For this review, take the finished solid that the model builds, in its own axes (mm). A direction names the side the tool comes from. Give positions to 0.01 mm unless a question says otherwise; leave off trailing zeros. Order: outer loops, then holes, each group sorted by start corner. A loop starts at its lowest first (then second) coordinate and runs counter-clockwise, first axis right, second up. Notation, with made-up numbers: (68.5, 9.5) - (94.5, 9.5) arc R31 ccw to (94.5, 44.5) - close; hole circle Ø7 at (35.25, 86.5). An arc over 180 degrees is marked (long way). Use a Markdown table: item, result. Add a question column.
1) Machinability: for faces 1 (the face through (3.451, 1.521, -6.645)), 2 (the face through (4, 0.8, -3)), which of the approach directions +Z, -Z, +X, -X, +Y, -Y give a long, thin tool a straight path to every point of the face, cutting with its end or side? Answer none if there is none.
2) We need section A-A on y = 2.7. Give the number of separate pieces and of enclosed holes in the cut face, then the cut area to 3 significant figures.
3) Clearance check with flat-ended pins moving along their axes: P1, Ø1.5, axis at y = 1, z = -6, coming from the -X side; P2, Ø2, axis at x = 3.5, z = -3.5, coming from the -Y side; P3, Ø1, axis at x = 4, y = 2.5, coming from the -Z side. State where each tip first meets the part, or that it passes through.
4) Wall thickness on L1, parallel to Y at x = 3, z = -3; L2, parallel to X at y = 0.3, z = -3.5; L3, parallel to X at y = 0.6, z = -4: over which ranges is each line inside the solid? List them lowest first.
5) We need section B-B on y = 0.45. Write out the cut boundary in (x, z) (3 decimals), then the cut area to 3 significant figures.
6) We need section C-C on z = -1.25. Write out the cut boundary in (x, y).
7) Mouldability with a two-part tool opening along X and no side actions: class faces 3 (the face through (2, 0, -5)), 4 (the face through (6.655, 1.479, -3.451)), 5 (the face through (4.041, 0.394, -5.217)), 6 (the face through (3.9, 2.6, -2.68)) as released by +X, released by -X, zero draft, split by the parting line, or undercut.
8) We need section D-D on y = 1.65. Write out the cut boundary in (x, z) (3 decimals), then the cut area to 3 significant figures.
```python
from build123d import *

# Parameters (mm, degrees)
SKETCH1_W           = 7
SKETCH1_H           = 7
BOSS_EXTRUDE1_DEPTH = 3
CUT_EXTRUDE1_DEPTH  = 7
CUT_EXTRUDE2_DEPTH  = 11
SKETCH4_R           = 1.8
CUT_EXTRUDE3_DEPTH  = 0.8
CUT_EXTRUDE4_DEPTH  = 0.4


with BuildPart() as part:
    # Sketch1 → Boss-Extrude1 (new body)
    with BuildSketch(Plane(origin=(0, 0, 0), x_dir=(1, 0, 0), z_dir=(0, 1, 0))):
        with Locations((3.5, 3.5)):
            Rectangle(SKETCH1_W, SKETCH1_H)
    extrude(amount=BOSS_EXTRUDE1_DEPTH)

    # Sketch2 → Cut-Extrude1 (cut)
    with BuildSketch(Plane.XY):
        Polygon((0, 0), (0.7, 3), (0, 3), align=None)
        Polygon((7, 0), (6.3, 3), (7, 3), align=None)
    extrude(amount=-CUT_EXTRUDE1_DEPTH, mode=Mode.SUBTRACT)

    # Sketch3 → Cut-Extrude2 (cut)
    with BuildSketch(Plane(origin=(0, 0, 0), x_dir=(0, 0, -1), z_dir=(1, 0, 0))):
        Polygon((0, 0), (0.7, 3), (0, 3), align=None)
        Polygon((7, 3), (6.3, 3), (7, 0), align=None)
    extrude(amount=CUT_EXTRUDE2_DEPTH, mode=Mode.SUBTRACT)

    # Sketch4 → Cut-Extrude3 (cut)
    with BuildSketch(Plane.XZ):
        with Locations(Location((3.5, -3.5, 0), (0, 0, 270))):
            Circle(SKETCH4_R)
    extrude(amount=-CUT_EXTRUDE3_DEPTH, mode=Mode.SUBTRACT)

    # Sketch6 → Cut-Extrude4 (cut)
    with BuildSketch(Plane(origin=(0, 3, 0), x_dir=(1, 0, 0), z_dir=(0, 1, 0))):
        with BuildLine():
            add(Edge.make_bspline(
                [(4.664072496, 2.366076672), (4.707347841, 2.33641431), (4.79406668, 2.276974329), (4.932000881, 2.200081193), (5.074319859, 2.130177652), (5.173227993, 2.092578566), (5.222866567, 2.073708884)],
                knots=[0, 0, 0, 0, 0.994855506, 1.99357661, 2.993045438, 4, 4, 4, 4], degree=3))
            Line((5.222866567, 2.073708884), (4.965554868, 1.58011914))
            add(Edge.make_bspline(
                [(4.965554868, 1.58011914), (4.912950568, 1.596402863), (4.806905677, 1.629229182), (4.706805134, 1.677225698), (4.656360157, 1.701413211)],
                knots=[0, 0, 0, 0, 0.992113803, 2, 2, 2, 2], degree=3))
            add(Edge.make_bspline(
                [(4.656360157, 1.701413211), (4.651410026, 1.703910751), (4.637075112, 1.711143291), (4.611037723, 1.728948088), (4.571310996, 1.752945912), (4.519597577, 1.786185947), (4.455377063, 1.827387082), (4.378441674, 1.876504864), (4.289852424, 1.934928076), (4.2261424, 1.976076602), (4.192217528, 1.99798773)],
                knots=[0, 0, 0, 0, 0.241377655, 0.698997227, 1.371388316, 2.263975901, 3.376788369, 4.695767198, 6.240533187, 8, 8, 8, 8], degree=3))
            add(Edge.make_bspline(
                [(4.192217528, 1.99798773), (4.164082126, 1.985938608), (4.107539341, 1.961723888), (4.019810769, 1.931906785), (3.929851311, 1.906788839), (3.83798057, 1.88548719), (3.743809701, 1.869659434), (3.647471832, 1.857521371), (3.548696902, 1.85040295), (3.481992412, 1.849703111), (3.448327304, 1.849349909)],
                knots=[0, 0, 0, 0, 0.961025642, 1.931341354, 2.907359807, 3.893838693, 4.891829695, 5.905170566, 6.942759923, 8, 8, 8, 8], degree=3))
            add(Edge.make_bspline(
                [(3.448327304, 1.849349909), (3.384469015, 1.850904143), (3.259644276, 1.853942228), (3.077633843, 1.87547395), (2.906612989, 1.912794393), (2.745831056, 1.96377118), (2.596254532, 2.030691184), (2.456571284, 2.111582166), (2.328715231, 2.208542848), (2.210924756, 2.318601555), (2.106714068, 2.44299724), (2.01548492, 2.579558487), (1.938201438, 2.727832608), (1.87588476, 2.888600431), (1.826634495, 3.060561995), (1.793056062, 3.244931239), (1.771444669, 3.440614719), (1.768994453, 3.575218022), (1.767738362, 3.644221704)],
                knots=[0, 0, 0, 0, 1.098101164, 2.146474535, 3.146072545, 4.104420533, 5.041773038, 5.958565538, 6.874115049, 7.795336865, 8.725215067, 9.658214839, 10.614563411, 11.594512188, 12.618591104, 13.685899083, 14.813688224, 16, 16, 16, 16], degree=3))
            add(Edge.make_bspline(
                [(1.767738362, 3.644221704), (1.768997302, 3.713222571), (1.771444596, 3.847355546), (1.7929084, 4.042662021), (1.827606571, 4.226372552), (1.876354652, 4.398607362), (1.939604685, 4.558913945), (2.017190294, 4.707202518), (2.10856287, 4.844051901), (2.214008903, 4.968173308), (2.331174894, 5.079358291), (2.459402401, 5.175598306), (2.597200561, 5.257768614), (2.745117273, 5.324625417), (2.903560867, 5.375574114), (3.071324913, 5.412775744), (3.249338156, 5.434570742), (3.371143561, 5.437560428), (3.433603746, 5.439093499)],
                knots=[0, 0, 0, 0, 1.193283781, 2.319662245, 3.393996131, 4.424093603, 5.411284417, 6.369670503, 7.313761776, 8.251713527, 9.181123148, 10.102053383, 11.01932051, 11.951118596, 12.903560284, 13.893239571, 14.919681386, 16, 16, 16, 16], degree=3))
            add(Edge.make_bspline(
                [(3.433603746, 5.439093499), (3.495615312, 5.437966268), (3.616563704, 5.435767699), (3.79292347, 5.412253487), (3.95956776, 5.376576627), (4.116694799, 5.325148401), (4.263499528, 5.258359333), (4.400745959, 5.177269062), (4.527633661, 5.081192592), (4.644198547, 4.971068574), (4.748454019, 4.847375423), (4.840809815, 4.712147514), (4.916635875, 4.563717786), (4.980514643, 4.404604546), (5.028132934, 4.233255975), (5.063284912, 4.050654395), (5.084451249, 3.856224461), (5.08696323, 3.722566855), (5.088251182, 3.654037409)],
                knots=[0, 0, 0, 0, 1.078752742, 2.104017338, 3.091035458, 4.041673215, 4.975566109, 5.892967701, 6.810684895, 7.740128604, 8.678185021, 9.621404646, 10.583875016, 11.573429805, 12.6009998, 13.674031063, 14.80742018, 16, 16, 16, 16], degree=3))
            add(Edge.make_bspline(
                [(5.088251182, 3.654037409), (5.086861856, 3.58175257), (5.084161048, 3.441232998), (5.060656035, 3.237166867), (5.02255362, 3.046054473), (4.983299325, 2.925957386), (4.964152625, 2.867378755)],
                knots=[0, 0, 0, 0, 1.083667057, 2.106616435, 3.076482036, 4, 4, 4, 4], degree=3))
            add(Edge.make_bspline(
                [(4.964152625, 2.867378755), (4.946989265, 2.824230782), (4.912073515, 2.73645404), (4.84305787, 2.609753708), (4.760943187, 2.484753896), (4.696820471, 2.406196533), (4.664072496, 2.366076672)],
                knots=[0, 0, 0, 0, 0.948216854, 1.928975575, 2.942311585, 4, 4, 4, 4], degree=3))
        make_face()
        with BuildLine():
            add(Edge.make_bspline(
                [(4.102473939, 2.726453275), (4.127780012, 2.754119398), (4.178452724, 2.809517857), (4.241114406, 2.90440552), (4.295822593, 3.006161549), (4.338835309, 3.117324632), (4.373428663, 3.236201997), (4.397571905, 3.363677482), (4.412566656, 3.499430632), (4.414289266, 3.592765315), (4.415174259, 3.640716095)],
                knots=[0, 0, 0, 0, 0.906820982, 1.815812261, 2.745108282, 3.70056618, 4.696560745, 5.740060838, 6.83895416, 8, 8, 8, 8], degree=3))
            add(Edge.make_bspline(
                [(4.415174259, 3.640716095), (4.414398079, 3.690052691), (4.412894495, 3.785625555), (4.400440515, 3.924411083), (4.378524584, 4.053416848), (4.349921684, 4.173180965), (4.310950729, 4.282734101), (4.263951968, 4.382902013), (4.208851462, 4.473931164), (4.144295177, 4.554319676), (4.073289316, 4.624992614), (3.997385018, 4.687424679), (3.915473431, 4.739684176), (3.827971743, 4.781723701), (3.735612195, 4.814802537), (3.638175965, 4.838817015), (3.53544327, 4.852870135), (3.465197405, 4.854784514), (3.429397016, 4.855760166)],
                knots=[0, 0, 0, 0, 1.335693338, 2.587451293, 3.768164612, 4.876224393, 5.916940853, 6.910477009, 7.867661778, 8.790666633, 9.694493319, 10.576027549, 11.446684429, 12.318352473, 13.199023277, 14.098364444, 15.030842682, 16, 16, 16, 16], degree=3))
            add(Edge.make_bspline(
                [(3.429397016, 4.855760166), (3.393356942, 4.854816175), (3.322865485, 4.852969805), (3.220031689, 4.838575915), (3.122373109, 4.815718183), (3.030128831, 4.782378038), (2.942464926, 4.740258761), (2.860247279, 4.688096064), (2.783487349, 4.626644322), (2.712123891, 4.556417609), (2.648385937, 4.476003653), (2.59172793, 4.38655956), (2.54488942, 4.287055852), (2.507276462, 4.178050834), (2.47721761, 4.060104683), (2.455571683, 3.932584455), (2.443101443, 3.795681707), (2.4415926, 3.701272351), (2.440815285, 3.652635166)],
                knots=[0, 0, 0, 0, 0.980107447, 1.917010591, 2.819119613, 3.703969481, 4.579773866, 5.459928929, 6.346604172, 7.250235365, 8.177620171, 9.131899985, 10.124404622, 11.161948974, 12.264485933, 13.431998172, 14.677033863, 16, 16, 16, 16], degree=3))
            add(Edge.make_bspline(
                [(2.440815285, 3.652635166), (2.441573469, 3.603294377), (2.44304577, 3.507480607), (2.45578752, 3.368559232), (2.476444238, 3.239125728), (2.505849447, 3.119233667), (2.543445207, 3.008746086), (2.589753063, 2.907816949), (2.64452751, 2.816572472), (2.707944858, 2.735840547), (2.77770996, 2.664816022), (2.852256943, 2.602898033), (2.930980725, 2.549856537), (3.014248538, 2.506760434), (3.102082714, 2.473663846), (3.194176957, 2.449777413), (3.291067215, 2.435539876), (3.35713374, 2.433648211), (3.390835317, 2.432683243)],
                knots=[0, 0, 0, 0, 1.356840463, 2.634818045, 3.833173645, 4.958776583, 6.025986406, 7.038359119, 8.007356852, 8.946032033, 9.855123386, 10.740685277, 11.607120956, 12.460971081, 13.313368256, 14.183325659, 15.073285775, 16, 16, 16, 16], degree=3))
            add(Edge.make_bspline(
                [(3.390835317, 2.432683243), (3.416109581, 2.433126684), (3.465894623, 2.43400017), (3.53944648, 2.443818905), (3.611093649, 2.458013111), (3.65736983, 2.472466064), (3.680398618, 2.479658403)],
                knots=[0, 0, 0, 0, 1.028828871, 2.026578908, 3.017950568, 4, 4, 4, 4], degree=3))
            add(Edge.make_bspline(
                [(3.680398618, 2.479658403), (3.645092364, 2.498106364), (3.575176857, 2.534638095), (3.467084084, 2.581186178), (3.358775331, 2.62312493), (3.28511213, 2.645783016), (3.248507593, 2.657042217)],
                knots=[0, 0, 0, 0, 1.021704821, 2.023239566, 3.017713044, 4, 4, 4, 4], degree=3))
            Line((3.248507593, 2.657042217), (3.444120573, 3.060888371))
            add(Edge.make_bspline(
                [(3.444120573, 3.060888371), (3.501325249, 3.041120096), (3.616286729, 3.001392746), (3.7823537, 2.92250788), (3.946106427, 2.832725945), (4.049959461, 2.762143896), (4.102473939, 2.726453275)],
                knots=[0, 0, 0, 0, 0.979271047, 1.967993817, 2.972492781, 4, 4, 4, 4], degree=3))
        make_face(mode=Mode.SUBTRACT)
    extrude(amount=-CUT_EXTRUDE4_DEPTH, mode=Mode.SUBTRACT)


solid = part.part
```
Checked values:
| question | item | result |
|---|---|---|
| 1 | face 1 | -Z, +X, -X, +Y |
| 1 | face 2 | -Y |
| 2 | separate pieces | 2 |
| 2 | enclosed holes | 1 |
| 2 | area | 26.4 mm² |
| 3 | P1 | x = 0.06 |
| 3 | P2 | y = 0.8 |
| 3 | P3 | z = -6.53 |
| 4 | L1 | 0.8 to 3 |
| 4 | L2 | 0.07 to 1.7, 5.3 to 6.93 |
| 4 | L3 | 0.14 to 1.77, 5.23 to 6.86 |
| 5 | outline | (0.105, -6.895) - (6.895, -6.895) - (6.895, -0.105) - (0.105, -0.105) - close; hole circle Ø3.6 at (3.5, -3.5) |
| 5 | area | 35.9 mm² |
| 6 | outline | (0, 0) - (7, 0) - (6.3, 3) - (0.7, 3) - close |
| 7 | face 3 | zero draft |
| 7 | face 4 | released by +X |
| 7 | face 5 | undercut |
| 7 | face 6 | undercut |
| 8 | outline | (0.385, -6.615) - (6.615, -6.615) - (6.615, -0.385) - (0.385, -0.385) - close |
| 8 | area | 38.8 mm² |
